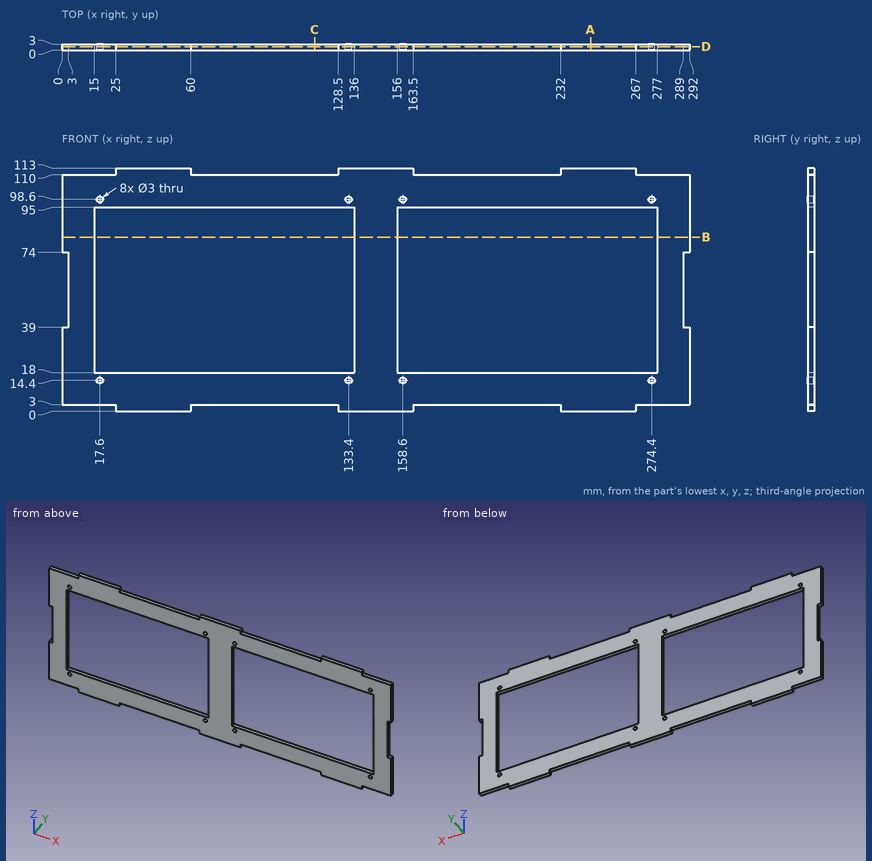
Part print with two shaded views. Sizes in mm from the minimum x, y, z corner. Coordinates: 2 decimals unless noted, no trailing zeros. Write each loop counter-clockwise with the first axis right and the second up, starting at its lowest first coordinate (ties: lowest second). Pieces come first, ordered by that corner, then holes.
1. Band-saw the part on B-B, the plane z = 81. Give the cut face in (x, y), and give its area (3 significant figures).
Answer block:
outline: (0, 0) - (15, 0) - (15, 3) - (0, 3) - close; (136, 0) - (156, 0) - (156, 3) - (136, 3) - close; (277, 0) - (292, 0) - (292, 3) - (277, 3) - close
area: 150 mm2
2. Band-saw the part on D-D, the plane y = 1.8. Give the number of separate pieces and of enclosed holes in the cut face, and give its area (3 significant figures).
Answer block:
separate pieces: 1
enclosed holes: 10
area: 13,000 mm2
3. Drop flat-ended pins along their axis: pin 1 (0.9 mm diameter, centred on x = 274, y = 1.5, fed in from -Z); pin 2 (1 mm diameter, centred on y = 2, z = 50, fed in from -X); pin 3 (0.9 mm diameter, centred on y = 1, z = 1, fed in from +X). Give the stop position or say it passes through.
Answer block:
pin 1: stops at z = 3
pin 2: stops at x = 3
pin 3: stops at x = 267
4. Band-saw the part on A-A, the plane x = 246. Give the cut face in (y, z), and give its area (3 significant figures).
Answer block:
outline: (0, 0) - (3, 0) - (3, 18) - (0, 18) - close; (0, 95) - (3, 95) - (3, 113) - (0, 113) - close
area: 108 mm2
5. Band-saw the part on C-C, the plane x = 117.5. Give the cut face in (y, z).
Answer block:
outline: (0, 3) - (3, 3) - (3, 18) - (0, 18) - close; (0, 95) - (3, 95) - (3, 110) - (0, 110) - close
6. Drill centre lines: probe 1 along Z at (x, y) = (133.4, 1.1); probe 2 along X at (y, z) = (1.8, 34); probe 3 along Z at (x, y) = (274.4, 1.9). Where is each one in solid material? Low to high.
Answer block:
probe 1: z = 0 to 12.9, 15.9 to 18, 95 to 97.1, 100.1 to 113
probe 2: x = 0 to 15, 136 to 156, 277 to 292
probe 3: z = 3 to 12.9, 15.9 to 18, 95 to 97.1, 100.1 to 110
